Geometry check sheet. Reference: the model listing, model coordinates, mm. Face numbers are marked on the shaded views. A direction names the side the tool comes from. Give positions to 0.01 mm unless a question says otherwise; leave off trailing zeros. Write each loop counter-clockwise with the first axis right and the second up, starting at its lowest first coordinate (ties: lowest second). Pieces come first, ordered by that corner, then holes. Notation, with made-up numbers: (21.25, -27.75) -> (71.25, -27.75) arc R25 cw to (71.25, 1.25) -> close; hole circle Ø4 at (25.25, 43). An arc over 180 degrees is marked (long way). Use a Markdown table: item, result. Add a question column.
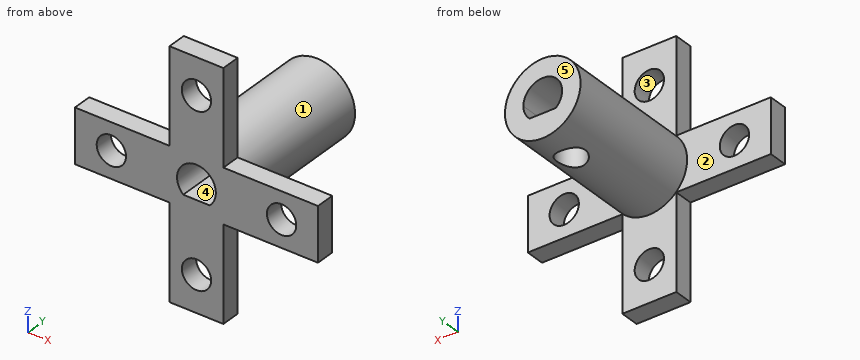
from build123d import *

# Parameters (mm, degrees)
SKETCH_1_W          = 25.7
SKETCH_1_H          = 5.7
SKETCH_1_R          = 1.55
SKETCH_1_W_2        = 5.7
SKETCH_1_H_2        = 25.7
EXTRUDE_1_DEPTH     = 2
SKETCH_2_R          = 4
EXTRUDE_2_DEPTH     = 15
CUT_EXTRUDE_1_DEPTH = 25.884633813
SKETCH_4_R          = 1.5
CUT_EXTRUDE_2_DEPTH = 26.691340954
CUT_EXTRUDE_START   = -1
SKETCH_5_R          = 1.5
CUT_EXTRUDE_3_DEPTH = 1


with BuildPart() as part:
    # 草图1 → 凸台-拉伸1 (new body)
    # profile 1 of 2: a face of its own
    with BuildSketch(Plane(origin=(0, 0, 0), x_dir=(1, 0, 0), z_dir=(0, 1, 0))):
        Rectangle(SKETCH_1_W, SKETCH_1_H)
        with Locations(Location((9, 0, 0), (0, 0, 270))):
            Circle(SKETCH_1_R, mode=Mode.SUBTRACT)
        with Locations(Location((-9, 0, 0), (0, 0, 270))):
            Circle(SKETCH_1_R, mode=Mode.SUBTRACT)
    # profile 2 of 2: a face of its own
    with BuildSketch(Plane(origin=(0, 0, 0), x_dir=(1, 0, 0), z_dir=(0, 1, 0))):
        Rectangle(SKETCH_1_W_2, SKETCH_1_H_2)
        with Locations(Location((0, 9, 0), (0, 0, 270))):
            Circle(SKETCH_1_R, mode=Mode.SUBTRACT)
        with Locations(Location((0, -9, 0), (0, 0, 270))):
            Circle(SKETCH_1_R, mode=Mode.SUBTRACT)
    extrude(amount=EXTRUDE_1_DEPTH)

    # 草图2 → 凸台-拉伸2 (add)
    with BuildSketch(Plane(origin=(0, 2, 0), x_dir=(1, 0, 0), z_dir=(0, 1, 0))):
        with Locations(Location((0, 0, 0), (0, 0, 270))):
            Circle(SKETCH_2_R)
    extrude(amount=EXTRUDE_2_DEPTH)

    # 草图3 → 切除-拉伸1 (cut, through all)
    with BuildSketch(Plane(origin=(0, 17, 0), x_dir=(1, 0, 0), z_dir=(0, 1, 0))):
        with BuildLine():
            Line((0, 1.5), (-1.397318861, 1.5))
            ThreePointArc((-1.397318861, 1.5), (-0.817923081, -1.879761111), (2.05, 0))
            ThreePointArc((2.05, 0), (1.879761111, 0.817923081), (1.397318861, 1.5))
            Line((1.397318861, 1.5), (0, 1.5))
        make_face()
    extrude(amount=-CUT_EXTRUDE_1_DEPTH, mode=Mode.SUBTRACT)

    # 草图4 → 切除-拉伸2 (cut, through all)
    with BuildSketch(Plane.XY.offset(-1.5)):
        with Locations(Location((0, 13, 0), (0, 0, 21.322909655))):
            Circle(SKETCH_4_R)
    extrude(amount=-CUT_EXTRUDE_2_DEPTH, mode=Mode.SUBTRACT)

    # 草图5 → 切除-拉伸3 (cut)
    with BuildSketch(Plane(origin=(0, 0, -1.5), x_dir=(-1, 0, 0), z_dir=(0, 0, -1)).offset(CUT_EXTRUDE_START)):
        with Locations(Location((0, 13, 0), (0, 0, 158.677090345))):
            Circle(SKETCH_5_R)
    extrude(amount=CUT_EXTRUDE_3_DEPTH, mode=Mode.SUBTRACT)


solid = part.part
1) Tool access check on the marked faces 4 and 5. Record the directions out of +Z, -Z, +X, -X, +Y, -Y that give a thin tool (end or side, any length) a straight path to the whole face; none if there is none.
2) Gauge pin test, flat ends, axial feed: P1, Ø0.6, axis at y = 1, z = 5.5, coming from the +X side; P2, Ø8, axis at x = -9.5, y = 5, coming from the -Z side; P3, Ø3, axis at x = 0, y = 14.5, coming from the +Z side; P4, Ø3, axis at x = 9, z = 0, coming from the -Y side. Record the tip position at first contact, or that the pin passes through.
3) Draft check along X on the marked faces 1, 2 and 3. Enter one of: +X half, -X half, draft (parallel to the pull), parting line (faces both ways), or undercut.
4) Sectioned sample at D-D, the plane y = 10. Enter the section's corners in (x, z).
5) Sectioned sample at C-C, the plane x = 0. Enter the section's corners in (y, z), and give its area (4 significant figures).
6) Material ranges on probe 1 along X at (y, z) = (1.15, 9); probe 2 along Y at (x, z) = (2.5, -4.5); probe 3 along Z at (x, y) = (0.75, 11), recorded low to high. Write a range as [from, to].
7) Sectioned sample at B-B, the plane z = 9. Enter the section's corners in (x, y).
8) Sectioned sample at A-A, the plane x = 9. Enter the section's corners in (y, z), and give its area (3 significant figures).
Check values:
| question | item | result |
|---|---|---|
| 1 | face 4 | +Y, -Y |
| 1 | face 5 | +Z, -Z, +X, -X, +Y |
| 2 | P1 | x = 2.85 |
| 2 | P2 | z = -2.85 |
| 2 | P3 | z = 4 |
| 2 | P4 | through |
| 3 | face 1 | parting line |
| 3 | face 2 | draft |
| 3 | face 3 | undercut |
| 4 | outline | circle Ø8 at (0, 0); hole (-1.4, -1.5) -> (1.4, -1.5) arc R2.05 ccw (long way) to start |
| 5 | outline | (0, -12.85) -> (2, -12.85) -> (2, -10.55) -> (0, -10.55) -> close; (0, -7.45) -> (2, -7.45) -> (2, -4) -> (11.5, -4) -> (11.5, -1.5) -> (0, -1.5) -> close; (0, 2.05) -> (17, 2.05) -> (17, 4) -> (2, 4) -> (2, 7.45) -> (0, 7.45) -> close; (0, 10.55) -> (2, 10.55) -> (2, 12.85) -> (0, 12.85) -> close; (14.5, -4) -> (17, -4) -> (17, -1.5) -> (14.5, -1.5) -> close |
| 5 | area | 91.15 mm² |
| 6 | probe 1 | [-2.85, -1.55], [1.55, 2.85] |
| 6 | probe 2 | [0, 2] |
| 6 | probe 3 | [-3.93, -1.5], [1.91, 3.93] |
| 7 | outline | (-2.85, 0) -> (-1.55, 0) -> (-1.55, 2) -> (-2.85, 2) -> close; (1.55, 0) -> (2.85, 0) -> (2.85, 2) -> (1.55, 2) -> close |
| 8 | outline | (0, -2.85) -> (2, -2.85) -> (2, -1.55) -> (0, -1.55) -> close; (0, 1.55) -> (2, 1.55) -> (2, 2.85) -> (0, 2.85) -> close |
| 8 | area | 5.20 mm² |
